from build123d import *

# Parameters (mm, degrees)
SKETCH1_R           = 6.35
BOSS_EXTRUDE1_DEPTH = 6.35
SKETCH2_R           = 38.1
BOSS_EXTRUDE2_DEPTH = 140.97
SKETCH3_R           = 6.35
BOSS_EXTRUDE3_DEPTH = 31.75
SKETCH4_R           = 12.7
BOSS_EXTRUDE4_DEPTH = 12.7
FILLET1_R           = 2.54
CUT_EXTRUDE1_DEPTH  = 2.54


with BuildPart() as part:
    # Sketch1 → Boss-Extrude1 (new body)
    with BuildSketch(Plane.XY):
        Circle(SKETCH1_R)
    extrude(amount=BOSS_EXTRUDE1_DEPTH)

    # Sketch2 → Boss-Extrude2 (add)
    with BuildSketch(Plane.XY.offset(6.35)):
        Circle(SKETCH2_R)
    extrude(amount=BOSS_EXTRUDE2_DEPTH)

    # Sketch3 → Boss-Extrude3 (add)
    with BuildSketch(Plane.XY.offset(147.32)):
        Circle(SKETCH3_R)
    extrude(amount=BOSS_EXTRUDE3_DEPTH)

    # Sketch4 → Boss-Extrude4 (add)
    with BuildSketch(Plane.XY.offset(179.07)):
        Circle(SKETCH4_R)
    extrude(amount=BOSS_EXTRUDE4_DEPTH)

    # Fillet1
    fillet1_edges = [part.edges().sort_by_distance(p)[0] for p in [
        (-6.35, 0, 179.07),
        (-12.7, 0, 179.07),
        (-12.7, 0, 191.77),
    ]]
    fillet(fillet1_edges, radius=FILLET1_R)

    # Sketch5 → Cut-Extrude1 (cut)
    with BuildSketch(Plane.XY.offset(191.77)):
        with BuildLine():
            Line((-0.475346185, 8.776619382), (0.540653815, 8.776619382))
            ThreePointArc((0.540653815, 8.776619382), (1.079469182, 8.55343475), (1.302653815, 8.014619382))
            Line((1.302653815, 8.014619382), (1.302653815, 1.918619382))
            ThreePointArc((1.302653815, 1.918619382), (1.525838448, 1.379804015), (2.064653815, 1.156619382))
            Line((2.064653815, 1.156619382), (8.160653815, 1.156619382))
            ThreePointArc((8.160653815, 1.156619382), (8.699469182, 0.93343475), (8.922653815, 0.394619382))
            Line((8.922653815, 0.394619382), (8.922653815, -0.621380618))
            ThreePointArc((8.922653815, -0.621380618), (8.699469182, -1.160195985), (8.160653815, -1.383380618))
            Line((8.160653815, -1.383380618), (2.064653815, -1.383380618))
            ThreePointArc((2.064653815, -1.383380618), (1.525838448, -1.60656525), (1.302653815, -2.145380618))
            Line((1.302653815, -2.145380618), (1.302653815, -8.241380618))
            ThreePointArc((1.302653815, -8.241380618), (1.079469182, -8.780195985), (0.540653815, -9.003380618))
            Line((0.540653815, -9.003380618), (-0.475346185, -9.003380618))
            ThreePointArc((-0.475346185, -9.003380618), (-1.014161552, -8.780195985), (-1.237346185, -8.241380618))
            Line((-1.237346185, -8.241380618), (-1.237346185, -2.145380618))
            ThreePointArc((-1.237346185, -2.145380618), (-1.460530818, -1.60656525), (-1.999346185, -1.383380618))
            Line((-1.999346185, -1.383380618), (-8.095346185, -1.383380618))
            ThreePointArc((-8.095346185, -1.383380618), (-8.634161552, -1.160195985), (-8.857346185, -0.621380618))
            Line((-8.857346185, -0.621380618), (-8.857346185, 0.394619382))
            ThreePointArc((-8.857346185, 0.394619382), (-8.634161552, 0.93343475), (-8.095346185, 1.156619382))
            Line((-8.095346185, 1.156619382), (-1.999346185, 1.156619382))
            ThreePointArc((-1.999346185, 1.156619382), (-1.460530818, 1.379804015), (-1.237346185, 1.918619382))
            Line((-1.237346185, 1.918619382), (-1.237346185, 8.014619382))
            ThreePointArc((-1.237346185, 8.014619382), (-1.014161552, 8.55343475), (-0.475346185, 8.776619382))
        make_face()
    extrude(amount=-CUT_EXTRUDE1_DEPTH, mode=Mode.SUBTRACT)


solid = part.part
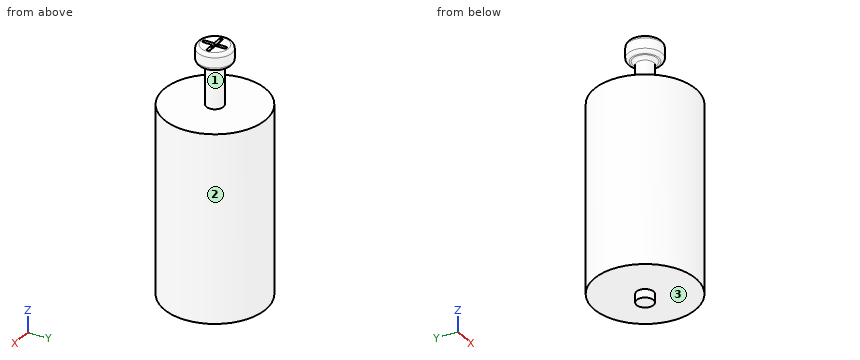
Work out the finished part from the listing and answer in its coordinate system (mm). Face numbers are marked on the shaded views. Round coordinates to 2 decimals unless told otherwise and drop trailing zeros. Write each loop counter-clockwise with the first axis right and the second up, starting at its lowest first coordinate (ties: lowest second). Pieces come first, ordered by that corner, then holes.
1) Straight lines are drawn through the part: line 1 (Z direction, x = -8.5, y = -3); line 2 (Y direction, x = -0.5, z = 119.5); line 3 (Z direction, x = 20, y = -30). For each, find the intervals that lie inside material, in ascending order.
2) A cutting plane is placed at B-B (x = -33). Give the vertices of the cut face in (y, z), plus the area to 3 significant figures.
3) A cutting plane is placed at D-D (z = 149.5). Give the vertices of the cut face in (x, y), plus the area to 3 significant figures.
4) A cutting plane is placed at C-C (y = -17.5). Give the vertices of the cut face in (x, z), plus the area to 3 significant figures.
5) A cutting plane is placed at A-A (z = 108.5). Give the vertices of the cut face in (x, y).
6) The mould has two halves that part along Z. Classify the marked faces 1, 2 and 3: pulls with the +Z half, pulls with the -Z half, needs draft (parallel to the pull), parting line crosses it, or undercut.
7) Given pin 1 Ø23 at (x, y) = (-18, -11) entering from -Z; pin 2 Ø2 at (y, z) = (25.5, 71.5) entering from -X; pin 3 Ø6 at (x, y) = (13, -22) entering from +Z, each flat-ended and moving along its own axis, determine where each tip first touches the part or whether it passes through.
Completed:
1. line 1: z = 6.35 to 147.32, 179.07 to 191.77
1. line 2: y = -38.1 to 38.1
1. line 3: z = 6.35 to 147.32
2. outline: (-19.04, 6.35) - (19.04, 6.35) - (19.04, 147.32) - (-19.04, 147.32) - close
2. area: 5,370 mm2
3. outline: circle Ø12.7 at (0, 0)
3. area: 127 mm2
4. outline: (-33.84, 6.35) - (33.84, 6.35) - (33.84, 147.32) - (-33.84, 147.32) - close
4. area: 9,540 mm2
5. outline: circle Ø76.2 at (0, 0)
6. face 1: undercut
6. face 2: needs draft
6. face 3: pulls with the -Z half
7. pin 1: stops at z = 6.35
7. pin 2: stops at x = -29.18
7. pin 3: stops at z = 147.32
